```python
from build123d import *

# Parameters (mm, degrees)
BOSS_EXTRUDE1_DEPTH       = 6.604
FILLET1_R                 = 6.35
F_4_CLEARANCE_HOLE1_D     = 3.2639
F_4_CLEARANCE_HOLE1_DEPTH = 9.652
F_4_CLEARANCE_HOLE1_TIP   = 0.980574487


with BuildPart() as part:
    # Sketch1 → Boss-Extrude1 (new body)
    with BuildSketch(Plane.XY):
        with BuildLine():
            Line((-6.35, -5.08), (-53.975, -5.08))
            Line((-53.975, -5.08), (-53.975, -17.78))
            ThreePointArc((-53.975, -17.78), (-24.613831362, -51.146124163), (18.36841389, -62.455547599))
            ThreePointArc((18.36841389, -62.455547599), (36.58027843, -57.005297746), (49.891818948, -43.434))
            Line((49.891818948, -43.434), (39.113266772, -37.211))
            ThreePointArc((39.113266772, -37.211), (0.611966481, -44.206961223), (0, -5.08))
            Line((0, -5.08), (-6.35, -5.08))
        make_face()
    extrude(amount=BOSS_EXTRUDE1_DEPTH)

    # Fillet1
    fillet1_edges = [part.edges().sort_by_distance(p)[0] for p in [
        (49.891818948, -43.434, 3.302),
    ]]
    fillet(fillet1_edges, radius=FILLET1_R)

    # #4 Clearance Hole1
    with Locations(Plane(origin=(-15.875, -11.43, 6.604), x_dir=(1, 0, 0), z_dir=(0, 0, 1))):
        with Locations((0, 0), (-25.4, 0)):
            Hole(F_4_CLEARANCE_HOLE1_D / 2, depth=F_4_CLEARANCE_HOLE1_DEPTH)
            with Locations((0, 0, -(F_4_CLEARANCE_HOLE1_DEPTH + F_4_CLEARANCE_HOLE1_TIP / 2))):  # 118° drill point
                Cone(0, F_4_CLEARANCE_HOLE1_D / 2, F_4_CLEARANCE_HOLE1_TIP, mode=Mode.SUBTRACT)


solid = part.part
```
For this review, take the finished solid that the model builds, in its own axes (mm). Coordinates: 2 decimals unless noted, no trailing zeros. Write each loop counter-clockwise with the first axis right and the second up, starting at its lowest first coordinate (ties: lowest second). Pieces come first, ordered by that corner, then holes. Notation, with made-up numbers: (27.25, 86.25) - (55.25, 86.25) arc R24 cw to (55.25, 105.25) - close; hole circle Ø5 at (42, 0). An arc over 180 degrees is marked (long way). Answer in a Markdown table with one row per item. Add a question column.
Q1. We need section B-B, the plane y = -11.43. State the section outline as (x, z) points (3 decimals).
Q2. For P1, Ø1.5, axis at x = 2.5, z = 5.5, coming from the +Y side; P2, Ø1, axis at y = -15.5, z = 4.5, coming from the +X side; P3, Ø2, axis at x = 34, z = 4, coming from the +Y side, all flat-tipped, find the tip position at first contact; note any pin that passes through.
Q3. We need section D-D, the plane y = -56. State the section outline as (x, z) points.
Q4. We need section C-C, the plane x = 11. State the section outline as (y, z) points.
Q5. For probe 1 along X at (y, z) = (-12.5, 5) (3 decimals); probe 2 along Y at (x, z) = (-39, 3.5); probe 3 along Y at (x, z) = (5, 3), list the stretches that pass through material, from the lowest coordinate up.
Q6. Draft analysis for pull direction Y (two halves, no side actions). For faces 1 (the cylindrical face through (-42.83, -10.94, 3.26)), 2 (the flat face through (-53.975, -11, 3)), 3 (the flat face through (41.508, -38.594, 3.256)), state which applies: +Y half, -Y half, draft (parallel to the pull), parting line (faces both ways), or undercut.
Q7. We need section A-A, the plane z = 2.75. State the section outline as (x, y) points (3 decimals).
Answer list:
| question | item | result |
|---|---|---|
| 1 | outline | (-53.975, 0) - (-42.907, 0) - (-42.907, 6.604) - (-53.975, 6.604) - close; (-39.643, 0) - (-17.507, 0) - (-17.507, 6.604) - (-39.643, 6.604) - close; (-14.243, 0) - (-5.247, 0) - (-5.247, 6.604) - (-14.243, 6.604) - close |
| 2 | P1 | stops at y = -45.09 |
| 2 | P2 | stops at x = -6.98 |
| 2 | P3 | stops at y = -42.56 |
| 3 | outline | (-15.4, 0) - (38.16, 0) - (38.16, 6.6) - (-15.4, 6.6) - close |
| 4 | outline | (-62.38, 0) - (-49.35, 0) - (-49.35, 6.6) - (-62.38, 6.6) - close |
| 5 | probe 1 | x = -53.975 to -42.507, -40.043 to -17.107, -14.643 to -5.839 |
| 5 | probe 2 | y = -39.65 to -5.08 |
| 5 | probe 3 | y = -61.8 to -47.11 |
| 6 | face 1 | undercut |
| 6 | face 2 | draft |
| 6 | face 3 | +Y half |
| 7 | outline | (-53.975, -17.78) arc R76.2 ccw to (18.368, -62.456) arc R38.1 ccw to (45.415, -49.648) arc R6.35 ccw to (43.837, -39.938) - (39.113, -37.211) arc R25.654 cw (long way) to (0, -5.08) - (-53.975, -5.08) - close; hole circle Ø3.264 at (-41.275, -11.43); hole circle Ø3.264 at (-15.875, -11.43) |
